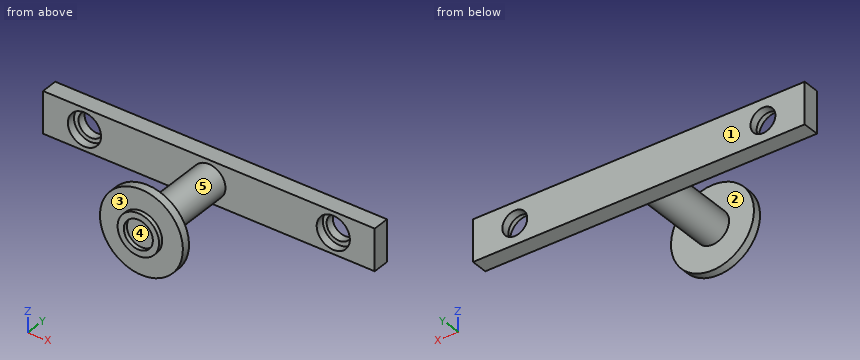
```python
from build123d import *

# Parameters (mm, degrees)
SKETCH2_R           = 5
BOSS_EXTRUDE1_DEPTH = 1
SKETCH3_R           = 2.5
SKETCH3_R_2         = 1.75
BOSS_EXTRUDE2_DEPTH = 0.5
SKETCH4_R           = 2
BOSS_EXTRUDE3_DEPTH = 10
SKETCH6_W           = 40
SKETCH6_H           = 5
BOSS_EXTRUDE4_DEPTH = 2
SKETCH9_R           = 2
CUT_EXTRUDE1_DEPTH  = 1
SKETCH10_R          = 1.5
CUT_EXTRUDE2_DEPTH  = 31


with BuildPart() as part:
    # Sketch2 → Boss-Extrude1 (new body)
    with BuildSketch(Plane(origin=(0, 0, 0), x_dir=(-1, 0, 0), z_dir=(0, 1, 0))):
        with Locations(Location((0, 0, 0), (0, 0, 90))):
            Circle(SKETCH2_R)
    extrude(amount=BOSS_EXTRUDE1_DEPTH)

    # Sketch3 → Boss-Extrude2 (add)
    with BuildSketch(Plane.XZ):
        with Locations(Location((0, 0, 0), (0, 0, 90))):
            Circle(SKETCH3_R)
        with Locations(Location((0, 0, 0), (0, 0, 270))):
            Circle(SKETCH3_R_2, mode=Mode.SUBTRACT)
    extrude(amount=BOSS_EXTRUDE2_DEPTH)

    # Sketch4 → Boss-Extrude3 (add)
    with BuildSketch(Plane(origin=(0, 1, 0), x_dir=(-1, 0, 0), z_dir=(0, 1, 0))):
        with Locations(Location((0, 0, 0), (0, 0, 90))):
            Circle(SKETCH4_R)
    extrude(amount=BOSS_EXTRUDE3_DEPTH)

    # Sketch6 → Boss-Extrude4 (add)
    with BuildSketch(Plane(origin=(0, 11, 0), x_dir=(-1, 0, 0), z_dir=(0, 1, 0))):
        Rectangle(SKETCH6_W, SKETCH6_H)
    extrude(amount=BOSS_EXTRUDE4_DEPTH)

    # Sketch9 → Cut-Extrude1 (cut)
    with BuildSketch(Plane.XZ.offset(-11)):
        with Locations(Location((-15, 0, 0), (0, 0, 270))):
            Circle(SKETCH9_R)
        with Locations(Location((15, 0, 0), (0, 0, 90))):
            Circle(SKETCH9_R)
    extrude(amount=-CUT_EXTRUDE1_DEPTH, mode=Mode.SUBTRACT)

    # Sketch10 → Cut-Extrude2 (cut)
    with BuildSketch(Plane.XZ.offset(-12)):
        with Locations(Location((-14.9595974, 0, 0), (0, 0, 270))):
            Circle(SKETCH10_R)
        with Locations(Location((14.9595974, 0, 0), (0, 0, 90))):
            Circle(SKETCH10_R)
    extrude(amount=-CUT_EXTRUDE2_DEPTH, mode=Mode.SUBTRACT)


solid = part.part
```
Check sheet for the modelled part. Datum: model origin and axes. Units: mm. Face numbers are marked on the shaded views. A direction names the side the tool comes from. Give positions to 0.01 mm unless a question says otherwise; leave off trailing zeros. Write each loop counter-clockwise with the first axis right and the second up, starting at its lowest first coordinate (ties: lowest second). Pieces come first, ordered by that corner, then holes.
Item 1: Cross-section at B-B (y = 8.5). Enter the section's corners in (x, z), and give its area (3 significant figures).
Item 2: Cross-section at D-D (z = 3.5). Enter the section's corners in (x, y).
Item 3: Cross-section at A-A (x = 0). Enter the section's corners in (y, z), and give its area (4 significant figures).
Item 4: Scan lines: L1, parallel to X at y = 12.65, z = 0; L2, parallel to X at y = 11.45, z = 0; L3, parallel to Y at x = 0.5, z = 2. Record each from-to range of solid material in increasing order.
Item 5: Access from +Z, -Z, +X, -X, +Y, -Y to the whole of each face (thin tool, end or side, straight path). Record for the marked faces 4 and 5.
Item 6: Draft check along Y on the marked faces 1, 2 and 3. Enter one of: released by +Y, released by -Y, zero draft, split by the parting line, or undercut.
Item 7: Cross-section at C-C (z = 0). Count the separate pieces of the cut face and the enclosed holes in it, and give its area (3 significant figures).
Item 8: Gauge pin test, flat ends, axial feed: pin 1 (1.5 mm diameter, centred on x = 9, z = 0.5, fed in from -Y); pin 2 (3 mm diameter, centred on y = 7.5, z = -4, fed in from +X); pin 3 (3.5 mm diameter, centred on x = 14.96, z = 0, fed in from -Y); pin 4 (4 mm diameter, centred on x = 1, z = -0.5, fed in from -Y). Record the tip position at first contact, or that the pin passes through.
Report:
1. outline: circle Ø4 at (0, 0)
1. area: 12.6 mm2
2. outline: (-3.57, 0) - (3.57, 0) - (3.57, 1) - (-3.57, 1) - close
3. outline: (-0.5, -2.5) - (0, -2.5) - (0, -5) - (1, -5) - (1, -2) - (11, -2) - (11, -2.5) - (13, -2.5) - (13, 2.5) - (11, 2.5) - (11, 2) - (1, 2) - (1, 5) - (0, 5) - (0, 2.5) - (-0.5, 2.5) - (-0.5, 1.75) - (0, 1.75) - (0, -1.75) - (-0.5, -1.75) - close
3. area: 60.75 mm2
4. L1: x = -20 to -16.46, -13.46 to 13.46, 16.46 to 20
4. L2: x = -20 to -17, -13 to 13, 17 to 20
4. L3: y = -0.5 to 1, 11 to 13
5. face 4: -Y
5. face 5: none
6. face 1: released by +Y
6. face 2: undercut
6. face 3: released by -Y
7. separate pieces: 3
7. enclosed holes: 0
7. area: 117 mm2
8. pin 1: stops at y = 11
8. pin 2: passes through
8. pin 3: stops at y = 12
8. pin 4: stops at y = -0.5
